Verification items for the finished model (mm, model axes). Round coordinates to 2 decimals unless told otherwise and drop trailing zeros. Write each loop counter-clockwise with the first axis right and the second up, starting at its lowest first coordinate (ties: lowest second). Pieces come first, ordered by that corner, then holes. Notation, with made-up numbers: (-29, -15) - (23, -15) arc R24 cw to (23, 10) - close; hole circle Ø2 at (33, 6.25). An arc over 180 degrees is marked (long way). Answer as a JSON object with one key per item and string values. Group by question number.
1) Thickness scan on line 1 (Z direction, x = -170.5, y = 4.75); line 2 (Z direction, x = -125.5, y = 4.3); line 3 (X direction, y = 0.6, z = -2124). Record the ranges inside material, lowest first.
2) Go/stop test with a flat-tipped pin: pin 1 Ø3.5 at (x, z) = (-146.14, -2124.39) entering from +Y. Record where the tip stops, or that it passes through.
3) Section check B-B (y = 3.8). Enter the section's corners in (x, z), then the cut area to 3 significant figures.
4) Section check A-A (x = -133). Enter the section's corners in (y, z).
```python
from build123d import *

# Parameters (mm, degrees)
SKETCH2_R                   = 1.5
SKETCH2_W                   = 16.6
SKETCH2_H                   = 5.13
BOSS_EXTRUDE1_DEPTH         = 5.13
F_1_2_CLEARANCE_HOLE1_D     = 13.89126
F_1_2_CLEARANCE_HOLE1_DEPTH = 5.13


with BuildPart() as part:
    # Sketch2 → Boss-Extrude1 (new body)
    with BuildSketch(Plane(origin=(0, 0, 0), x_dir=(1, 0, 0), z_dir=(0, 1, 0))):
        with BuildLine():
            Line((-210.314103066, 2127.521742865), (-210.314103066, 2196.481742865))
            ThreePointArc((-210.314103066, 2196.481742865), (-206.594359187, 2205.461998986), (-197.614103066, 2209.181742865))
            Line((-197.614103066, 2209.181742865), (-99.314103066, 2209.181742865))
            ThreePointArc((-99.314103066, 2209.181742865), (-98.606996285, 2208.888849646), (-98.314103066, 2208.181742865))
            Line((-98.314103066, 2208.181742865), (-98.314103066, 2115.821742865))
            ThreePointArc((-98.314103066, 2115.821742865), (-98.606996285, 2115.114636084), (-99.314103066, 2114.821742865))
            Line((-99.314103066, 2114.821742865), (-197.614103066, 2114.821742865))
            ThreePointArc((-197.614103066, 2114.821742865), (-206.594359187, 2118.541486744), (-210.314103066, 2127.521742865))
        make_face()
        with Locations((-146.144103066, 2199.616742865)):
            Circle(SKETCH2_R, mode=Mode.SUBTRACT)
        with Locations((-146.144103066, 2124.386742865)):
            Circle(SKETCH2_R, mode=Mode.SUBTRACT)
        with Locations((-129.544103066, 2124.326494276)):
            Rectangle(SKETCH2_W, SKETCH2_H, mode=Mode.SUBTRACT)
        with Locations((-162.744103066, 2124.386742865)):
            Rectangle(SKETCH2_W, SKETCH2_H, mode=Mode.SUBTRACT)
        with Locations((-162.744103066, 2199.615933693)):
            Rectangle(SKETCH2_W, SKETCH2_H, mode=Mode.SUBTRACT)
        with Locations((-129.544103066, 2199.555685104)):
            Rectangle(SKETCH2_W, SKETCH2_H, mode=Mode.SUBTRACT)
    extrude(amount=BOSS_EXTRUDE1_DEPTH)

    # 1/2 Clearance Hole1
    with Locations(Plane(origin=(0, 5.13, 0), x_dir=(-1, 0, 0), z_dir=(0, 1, 0))):
        with Locations((-8.273522926, -2159.461742865)):
            Hole(F_1_2_CLEARANCE_HOLE1_D / 2, depth=F_1_2_CLEARANCE_HOLE1_DEPTH)


solid = part.part
```
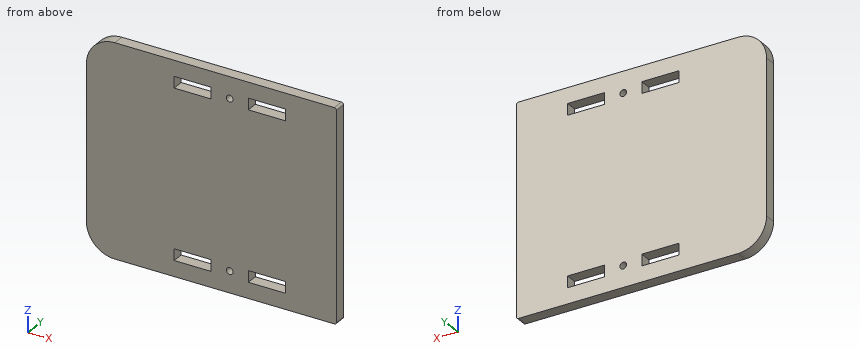
Returned:
{
 "1": {"line 1": "-2209.18 to -2202.18, -2197.05 to -2126.95, -2121.82 to -2114.82", "line 2": "-2209.18 to -2202.12, -2196.99 to -2126.89, -2121.76 to -2114.82", "line 3": "-209.82 to -171.04, -154.44 to -147.59, -144.69 to -137.84, -121.24 to -98.31"},
 "2": {"pin 1": "y = 5.13"},
 "3": {"outline": "(-210.31, -2196.48) arc R12.7 ccw to (-197.61, -2209.18) - (-99.31, -2209.18) arc R1 ccw to (-98.31, -2208.18) - (-98.31, -2115.82) arc R1 ccw to (-99.31, -2114.82) - (-197.61, -2114.82) arc R12.7 ccw to (-210.31, -2127.52) - close; hole (-171.04, -2202.18) - (-154.44, -2202.18) - (-154.44, -2197.05) - (-171.04, -2197.05) - close; hole (-171.04, -2126.95) - (-154.44, -2126.95) - (-154.44, -2121.82) - (-171.04, -2121.82) - close; hole circle Ø3 at (-146.14, -2199.62); hole circle Ø3 at (-146.14, -2124.39); hole (-137.84, -2202.12) - (-121.24, -2202.12) - (-121.24, -2196.99) - (-137.84, -2196.99) - close; hole (-137.84, -2126.89) - (-121.24, -2126.89) - (-121.24, -2121.76) - (-137.84, -2121.76) - close", "area": "10,100 mm2"},
 "4": {"outline": "(0, -2209.18) - (5.13, -2209.18) - (5.13, -2202.12) - (0, -2202.12) - close; (0, -2196.99) - (5.13, -2196.99) - (5.13, -2126.89) - (0, -2126.89) - close; (0, -2121.76) - (5.13, -2121.76) - (5.13, -2114.82) - (0, -2114.82) - close"}
}
